Build history of the part. All positions in model axes, mm. Face numbers are marked on the shaded views. A direction names the side the tool comes from. Give positions to 0.01 mm unless a question says otherwise; leave off trailing zeros. Order: outer loops, then holes, each group sorted by start corner. A loop starts at its lowest first (then second) coordinate and runs counter-clockwise, first axis right, second up. Notation, with made-up numbers: (6, -14) - (51, -14) arc R27 ccw to (51, 13) - close; hole circle Ø4 at (57.25, 81). An arc over 180 degrees is marked (long way). Use a Markdown table: item, result.
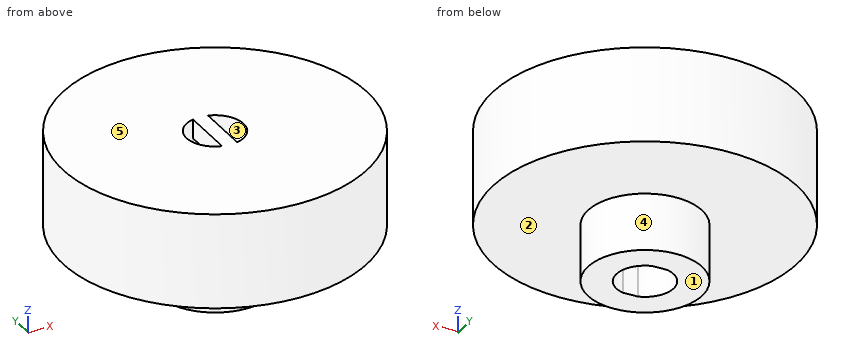
from build123d import *

# Parameters (mm, degrees)
SKETCH1_R               = 25.4
BOSS_EXTRUDE1_DEPTH     = 15.875
SKETCH6_R               = 9.525
BOSS_EXTRUDE3_DEPTH     = 9.525
CUT_EXTRUDE3_DEPTH      = 49.09113031
CUT_EXTRUDE3_DEPTH_BACK = 49.09113031
CUT_EXTRUDE5_DEPTH      = 22.225


with BuildPart() as part:
    # Sketch1 → Boss-Extrude1 (new body)
    with BuildSketch(Plane.XY):
        with Locations((-6.575565897, 0)):
            Circle(SKETCH1_R)
    extrude(amount=BOSS_EXTRUDE1_DEPTH)

    # Sketch6 → Boss-Extrude3 (add)
    with BuildSketch(Plane(origin=(0, 0, 0), x_dir=(-1, 0, 0), z_dir=(0, 0, -1))):
        with Locations(Location((6.575565897, 0, 0), (0, 0, 180))):
            Circle(SKETCH6_R)
    extrude(amount=BOSS_EXTRUDE3_DEPTH)

    # Sketch2 → Cut-Extrude3 (cut, two sides: drawn at the far end of the back side and taken through both)
    with BuildSketch(Plane.XY.offset(15.875).offset(-CUT_EXTRUDE3_DEPTH_BACK)):
        with BuildLine():
            Line((-7.824241479, 4.595891159), (-7.824241479, -4.595891159))
            ThreePointArc((-7.824241479, -4.595891159), (-11.338065897, 0), (-7.824241479, 4.595891159))
        make_face()
        with BuildLine():
            Line((-5.305565897, 4.590044254), (-5.305565897, -4.590044254))
            ThreePointArc((-5.305565897, -4.590044254), (-1.813065897, 0), (-5.305565897, 4.590044254))
        make_face()
    extrude(amount=CUT_EXTRUDE3_DEPTH + CUT_EXTRUDE3_DEPTH_BACK, mode=Mode.SUBTRACT)

    # Sketch10 → Cut-Extrude5 (cut)
    with BuildSketch(Plane(origin=(0, 0, -9.525), x_dir=(-1, 0, 0), z_dir=(0, 0, -1))):
        Polygon((5.305565897, 4.590044254), (5.305565897, -4.590044254), (7.824241479, -4.595891159), (7.824241479, 4.595891159), align=None)
    extrude(amount=-CUT_EXTRUDE5_DEPTH, mode=Mode.SUBTRACT)


solid = part.part
1) Two-plate mould, pull along Y, no slides. Class the marked faces 3, 4 and 5: +Y half, -Y half, draft (parallel to the pull), parting line (faces both ways), or undercut.
Computed:
| item | result |
|---|---|
| face 3 | undercut |
| face 4 | parting line |
| face 5 | draft |
2) Tool access for the marked faces 1 and 2: list every direction of +Z, -Z, +X, -X, +Y, -Y with a clear straight run to the whole face (end or side of a thin tool).
Computed:
| item | result |
|---|---|
| face 1 | -Z, +X, -X, +Y, -Y |
| face 2 | -Z |
3) Wall check: line 1 (Z direction, x = -11, y = -14) (3 decimals); line 2 (Y direction, x = -7, z = -3); line 3 (Y direction, x = -4.5, z = -3.5). Give the ranges that are in metal, low to high. Write a range as from..to.
Computed:
| item | result |
|---|---|
| line 1 | z = 0..15.875 |
| line 2 | y = -9.52..-4.59, 4.59..9.52 |
| line 3 | y = -9.3..-4.29, 4.29..9.3 |
4) Slice it at D-D (z = 6.5). Write the cut outline in (x, y) (1 decimal).
Computed:
| item | result |
|---|---|
| outline | circle Ø50.8 at (-6.6, 0); hole (-7.8, -4.6) - (-5.3, -4.6) arc R4.8 ccw to (-5.3, 4.6) - (-7.8, 4.6) arc R4.8 ccw to start |
5) Pin check, flat tips, straight feed: P1, Ø12, axis at x = -22.5, z = 4.5, coming from the -Y side; P2, Ø6, axis at x = -8.5, y = 17, coming from the -Z side; P3, Ø2, axis at x = -7, y = -1, coming from the -Z side; P4, Ø10, axis at y = 17, z = -6.5, coming from the +X side. Stop position of each tip, or through.
Computed:
| item | result |
|---|---|
| P1 | stops at y = -23.38 |
| P2 | stops at z = 0 |
| P3 | stops at z = 12.7 |
| P4 | passes through |
6) Slice it at C-C (x = 1). Write the cut outline in (y, z) (3 decimals).
Computed:
| item | result |
|---|---|
| outline | (-24.244, 0) - (-5.774, 0) - (-5.774, -9.525) - (5.774, -9.525) - (5.774, 0) - (24.244, 0) - (24.244, 15.875) - (-24.244, 15.875) - close |
7) Slice it at A-A (y = 0). Write the cut outline in (x, z) (3 decimals), and give its area (3 significant figures).
Computed:
| item | result |
|---|---|
| outline | (-31.976, 0) - (-16.101, 0) - (-16.101, -9.525) - (-11.338, -9.525) - (-11.338, 15.875) - (-31.976, 15.875) - close; (-7.824, 12.7) - (-5.306, 12.7) - (-5.306, 15.875) - (-7.824, 15.875) - close; (-1.813, -9.525) - (2.949, -9.525) - (2.949, 0) - (18.824, 0) - (18.824, 15.875) - (-1.813, 15.875) - close |
| area | 754 mm² |
